Source: CAD feature listing. Evaluate the final solid. Frame: model axes, mm. Face numbers are marked on the shaded views. A direction names the side the tool comes from. Round coordinates to 2 decimals unless told otherwise and drop trailing zeros. Loops run counter-clockwise (first coordinate to the right, second up) from the corner with the lowest first, then second, coordinate; pieces in that order, holes last.
(1) Section C-C, the plane x = 1. Return the cut outline in (y, z).
(2) Section A-A, the plane y = 0.25. Return the cut outline in (x, z).
(3) Section B-B, the plane z = 8.5. Return the cut outline in (x, y), plus the area to 3 significant figures.
(4) Material intervals for probe 1 along Y at (x, z) = (10.5, 1.5); probe 2 along Y at (x, z) = (2, 3.25); probe 3 along X at (y, z) = (2.75, 7.25), sorted ascending.
(5) Mould query, pull axis Y, two halves, no side actions, for the marked faces 1, 2, 3 and 4. Classes: pulls with the +Y half, pulls with the -Y half, needs draft (parallel to the pull), parting line crosses it, or undercut.
(6) Section D-D, the plane y = 7. Return the cut outline in (x, z).
(7) Set-up query: the marked faces 5, 6 and 7. Return all of +Z, -Z, +X, -X, +Y, -Y with unobstructed straight access to the full face (end or side cutting, diameter ignored); none if empty.
(8) First-contact query: pin 1 Ø3 at (x, z) = (-14.5, 4) entering from +Y; pin 2 Ø2 at (x, z) = (14.5, 9) entering from +Y; pin 3 Ø1 at (x, z) = (-13.5, 10.5) entering from +Y; pin 4 Ø1 at (y, z) = (5, 4.5) entering from -X. Flat tips, straight axial feed; report the tip coordinate or a pass-through.
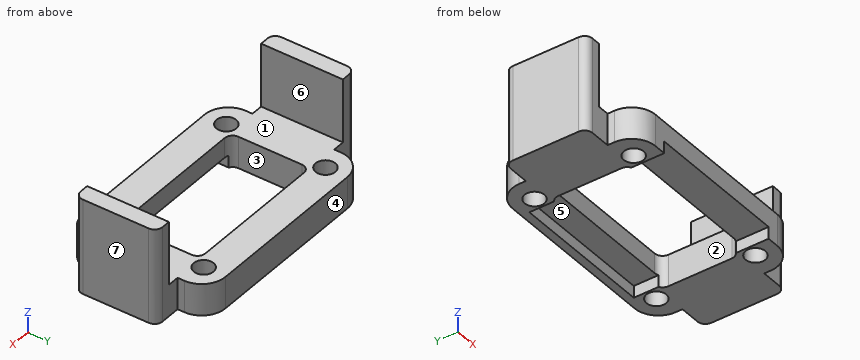
```python
from build123d import *

# Parameters (mm, degrees)
F0_R     = 1.25
F1_DEPTH = 4
F2_W     = 18
F2_H     = 17
F3_DEPTH = 1.5
F5_DEPTH = 8


with BuildPart() as f1:
    # F0 (on Top) → F1 (new body)
    with BuildSketch(Plane.XY):
        with BuildLine():
            Line((-10.5, -9), (10.5, -9))
            ThreePointArc((10.5, -9), (12.62132, -8.12132), (13.5, -6))
            Line((13.5, -6), (13.5, -5.154641))
            Line((13.5, -5.154641), (13.5, 5.154641))
            Line((13.5, 5.154641), (13.5, 6))
            ThreePointArc((13.5, 6), (12.62132, 8.12132), (10.5, 9))
            Line((10.5, 9), (-10.5, 9))
            ThreePointArc((-10.5, 9), (-12.62132, 8.12132), (-13.5, 6))
            Line((-13.5, 6), (-13.5, 5.154641))
            Line((-13.5, 5.154641), (-13.5, -5.154641))
            Line((-13.5, -5.154641), (-13.5, -6))
            ThreePointArc((-13.5, -6), (-12.62132, -8.12132), (-10.5, -9))
        make_face()
        with Locations((-10.5, -6.25)):
            Circle(F0_R, mode=Mode.SUBTRACT)
        with Locations((10.5, -6.25)):
            Circle(F0_R, mode=Mode.SUBTRACT)
        with Locations((-10.5, 6.25)):
            Circle(F0_R, mode=Mode.SUBTRACT)
        with BuildLine():
            ThreePointArc((9.5, -4), (9.207107, -4.707107), (8.5, -5))
            Line((8.5, -5), (-8.5, -5))
            ThreePointArc((-8.5, -5), (-9.207107, -4.707107), (-9.5, -4))
            Line((-9.5, -4), (-9.5, 4))
            ThreePointArc((-9.5, 4), (-9.207107, 4.707107), (-8.5, 5))
            Line((-8.5, 5), (8.5, 5))
            ThreePointArc((8.5, 5), (9.207107, 4.707107), (9.5, 4))
            Line((9.5, 4), (9.5, -4))
        make_face(mode=Mode.SUBTRACT)
        with Locations((10.5, 6.25)):
            Circle(F0_R, mode=Mode.SUBTRACT)
        with BuildLine():
            Line((13.5, 5.154641), (13.5, -5.154641))
            Line((13.5, -5.154641), (16.1, -5.154641))
            ThreePointArc((16.1, -5.154641), (16.807107, -4.861748), (17.1, -4.154641))
            Line((17.1, -4.154641), (17.1, 4.154641))
            ThreePointArc((17.1, 4.154641), (16.807107, 4.861748), (16.1, 5.154641))
            Line((16.1, 5.154641), (13.5, 5.154641))
        make_face()
        with BuildLine():
            Line((-16.1, -5.154641), (-13.5, -5.154641))
            Line((-13.5, -5.154641), (-13.5, 5.154641))
            Line((-13.5, 5.154641), (-16.1, 5.154641))
            ThreePointArc((-16.1, 5.154641), (-16.807107, 4.861748), (-17.1, 4.154641))
            Line((-17.1, 4.154641), (-17.1, -4.154641))
            ThreePointArc((-17.1, -4.154641), (-16.807107, -4.861748), (-16.1, -5.154641))
        make_face()
    extrude(amount=F1_DEPTH)

    # F2 (on face) → F3 (cut)
    with BuildSketch(Plane(origin=(0, 0, 0), x_dir=(1, 0, 0), z_dir=(0, 0, -1))):
        with Locations((0, 0.5)):
            Rectangle(F2_W, F2_H)
    extrude(amount=-F3_DEPTH, mode=Mode.SUBTRACT)

    # F4 (on face) → F5 (join)
    with BuildSketch(Plane.XY.offset(4)):
        with BuildLine():
            ThreePointArc((-16.1, 5.154641), (-16.807107, 4.861748), (-17.1, 4.154641))
            Line((-17.1, 4.154641), (-17.1, -4.154641))
            ThreePointArc((-17.1, -4.154641), (-16.807107, -4.861748), (-16.1, -5.154641))
            Line((-16.1, -5.154641), (-15, -5.154641))
            Line((-15, -5.154641), (-15, 5.154641))
            Line((-15, 5.154641), (-16.1, 5.154641))
        make_face()
        with BuildLine():
            ThreePointArc((17.1, 4.154641), (16.807107, 4.861748), (16.1, 5.154641))
            Line((16.1, 5.154641), (15, 5.154641))
            Line((15, 5.154641), (15, -5.154641))
            Line((15, -5.154641), (16.1, -5.154641))
            ThreePointArc((16.1, -5.154641), (16.807107, -4.861748), (17.1, -4.154641))
            Line((17.1, -4.154641), (17.1, 4.154641))
        make_face()
    extrude(amount=F5_DEPTH)


solid = f1.part
```
Output values:
1. outline: (-9, 1.5) - (-5, 1.5) - (-5, 4) - (-9, 4) - close; (5, 1.5) - (8, 1.5) - (8, 0) - (9, 0) - (9, 4) - (5, 4) - close
2. outline: (-17.1, 0) - (-9.5, 0) - (-9.5, 4) - (-15, 4) - (-15, 12) - (-17.1, 12) - close; (9.5, 0) - (17.1, 0) - (17.1, 12) - (15, 12) - (15, 4) - (9.5, 4) - close
3. outline: (-17.1, -4.15) arc R1 ccw to (-16.1, -5.15) - (-15, -5.15) - (-15, 5.15) - (-16.1, 5.15) arc R1 ccw to (-17.1, 4.15) - close; (15, -5.15) - (16.1, -5.15) arc R1 ccw to (17.1, -4.15) - (17.1, 4.15) arc R1 ccw to (16.1, 5.15) - (15, 5.15) - close
3. area: 42.4 mm2
4. probe 1: y = -9 to -7.5, -5 to 5, 7.5 to 9
4. probe 2: y = -9 to -5, 5 to 9
4. probe 3: x = -17.1 to -15, 15 to 17.1
5. face 1: needs draft
5. face 2: undercut
5. face 3: undercut
5. face 4: pulls with the +Y half
6. outline: (-13.33, 0) - (-11.5, 0) - (-11.5, 4) - (-13.33, 4) - close; (-9.5, 0) - (-9, 0) - (-9, 1.5) - (9, 1.5) - (9, 0) - (9.5, 0) - (9.5, 4) - (-9.5, 4) - close; (11.5, 0) - (13.33, 0) - (13.33, 4) - (11.5, 4) - close
7. face 5: -Z, -Y
7. face 6: +Z, +Y, -Y
7. face 7: +Z, -Z, +X, +Y, -Y
8. pin 1: stops at y = 7.66
8. pin 2: stops at y = 5.15
8. pin 3: passes through
8. pin 4: stops at x = -17.04
